from build123d import *

# Parameters (mm, degrees)
BOSS_EXTRUDE1_DEPTH     = 3
CUT_EXTRUDE4_DEPTH      = 13.469963913
CUT_EXTRUDE4_DEPTH_BACK = 13.469963913
CUT_EXTRUDE5_DEPTH      = 12.324751653
CUT_EXTRUDE5_DEPTH_BACK = 12.324751653
SKETCH6_R               = 18.5
FILLET1_R               = 0.5


with BuildPart() as part:
    # Sketch1 → Boss-Extrude1 (new, symmetric)
    with BuildSketch(Plane.XY):
        Polygon((-6, -1), (6, -1), (6, 1), (3.5, 1), (3.5, 7.5), (1.5, 7.5), (1.5, 1), (-1.5, 1), (-1.5, 7.5), (-3.5, 7.5), (-3.5, 1), (-6, 1), align=None)
    extrude(amount=BOSS_EXTRUDE1_DEPTH, both=True)

    # Sketch5 → Cut-Extrude4 (cut, two sides: drawn at the far end of the back side and taken through both)
    with BuildSketch(Plane.ZY.offset(3.5).offset(-CUT_EXTRUDE4_DEPTH_BACK)):
        with BuildLine():
            Line((1.25, 4.5), (-1.25, 4.5))
            ThreePointArc((-1.25, 4.5), (-2.25, 5.5), (-1.25, 6.5))
            Line((-1.25, 6.5), (1.25, 6.5))
            ThreePointArc((1.25, 6.5), (2.25, 5.5), (1.25, 4.5))
        make_face()
    extrude(amount=CUT_EXTRUDE4_DEPTH + CUT_EXTRUDE4_DEPTH_BACK, mode=Mode.SUBTRACT)

    # Sketch6 → Cut-Extrude5 (cut, two sides: drawn at the far end of the back side and taken through both)
    with BuildSketch(Plane.XY.offset(3).offset(-CUT_EXTRUDE5_DEPTH_BACK)):
        with Locations((0, -18.5)):
            Circle(SKETCH6_R)
        with BuildLine():
            Line((-6, 1), (-3.5, 1))
            ThreePointArc((-3.5, 1), (-4.760065757, 0.731270733), (-6, 0.381207588))
            Line((-6, 0.381207588), (-6, 1))
        make_face()
        with BuildLine():
            Line((3.5, 1), (6, 1))
            Line((6, 1), (6, 0.381207588))
            ThreePointArc((6, 0.381207588), (4.760065757, 0.731270733), (3.5, 1))
        make_face()
    extrude(amount=CUT_EXTRUDE5_DEPTH + CUT_EXTRUDE5_DEPTH_BACK, mode=Mode.SUBTRACT)

    # Fillet1
    fillet1_edges = [part.edges().sort_by_distance(p)[0] for p in [
        (6, -1, 0),
        (-6, -1, 0),
    ]]
    fillet(fillet1_edges, radius=FILLET1_R)


solid = part.part
Design review of the part built by this model. Coordinates are the model's own, in mm. A direction names the side the tool comes from. Coordinates: 2 decimals unless noted, no trailing zeros. Loops run counter-clockwise (first coordinate to the right, second up) from the corner with the lowest first, then second, coordinate; pieces in that order, holes last.
Item 1: Add section A-A (z = 0.15). Write out the cut boundary in (x, y), and give its area (3 significant figures).
Completed:
outline: (-6, -0.31) arc R0.5 ccw to (-5.36, -0.79) arc R18.5 cw to (5.36, -0.79) arc R0.5 ccw to (6, -0.31) - (6, 0.38) arc R19.81 ccw to (3.5, 1) - (3.5, 4.5) - (1.5, 4.5) - (1.5, 1) - (-1.5, 1) - (-1.5, 4.5) - (-3.5, 4.5) - (-3.5, 1) arc R19.81 ccw to (-6, 0.38) - close; (-3.5, 6.5) - (-1.5, 6.5) - (-1.5, 7.5) - (-3.5, 7.5) - close; (1.5, 6.5) - (3.5, 6.5) - (3.5, 7.5) - (1.5, 7.5) - close
area: 32.3 mm2
Item 2: Wall thickness on L1, parallel to X at y = 1.5, z = 2.1; L2, parallel to Y at x = -3.25, z = 1.95; L3, parallel to Y at x = -0.25, z = 2.65: over which ranges is each line inside the solid? List them lowest first.
Completed:
L1: x = -3.5 to -1.5, 1.5 to 3.5
L2: y = -0.29 to 4.79, 6.21 to 7.5
L3: y = 0 to 1
Item 3: Add section D-D (x = -2.5). Write out the cut boundary in (y, z).
Completed:
outline: (-0.17, -3) - (7.5, -3) - (7.5, 3) - (-0.17, 3) - close; hole (4.5, -1.25) arc R1 ccw to (6.5, -1.25) - (6.5, 1.25) arc R1 ccw to (4.5, 1.25) - close
Item 4: Clearance check with flat-ended pins moving along their axes: pin 1 (1.6 mm diameter, centred on x = 3, z = 0, fed in from -Y); pin 2 (1 mm diameter, centred on x = -2.5, z = 0.5, fed in from -Y); pin 3 (0.9 mm diameter, centred on x = 0.5, z = 1, fed in from +Y). State where each tip first meets the part, or that it passes through.
Completed:
pin 1: stops at y = -0.39
pin 2: stops at y = -0.24
pin 3: stops at y = 1
Item 5: Draft analysis for pull direction Z (two halves, no side actions). For faces 4 (the cylindrical face through (-2.49, 5.52, 2.25)), 5 (the flat face through (2, 2, 3)), 6 (the flat face through (-3.5, 4, 0)), state which applies: pulls with the +Z half, pulls with the -Z half, needs draft (parallel to the pull), parting line crosses it, or undercut.
Completed:
face 4: undercut
face 5: pulls with the +Z half
face 6: needs draft
Item 6: For faces 1 (the flat face through (0, 1, 0)), 2 (the flat face through (3.5, 3, 0)), 3 (the flat face through (3, 6.5, 0)), list the 3-axis set-ups (+Z, -Z, +X, -X, +Y, -Y) from which the entire face can be reached by the end or side of a thin tool; tool diameter is ignored.
Completed:
face 1: +Z, -Z, +Y
face 2: +Z, -Z, +X, +Y
face 3: +X, -X
Item 7: Add section B-B (y = 3). Write out the cut boundary in (x, z).
Completed:
outline: (-3.5, -3) - (-1.5, -3) - (-1.5, 3) - (-3.5, 3) - close; (1.5, -3) - (3.5, -3) - (3.5, 3) - (1.5, 3) - close
Item 8: Add section C-C (y = 5.5). Write out the cut boundary in (x, z), and give its area (3 significant figures).
Completed:
outline: (-3.5, -3) - (-1.5, -3) - (-1.5, -2.25) - (-3.5, -2.25) - close; (-3.5, 2.25) - (-1.5, 2.25) - (-1.5, 3) - (-3.5, 3) - close; (1.5, -3) - (3.5, -3) - (3.5, -2.25) - (1.5, -2.25) - close; (1.5, 2.25) - (3.5, 2.25) - (3.5, 3) - (1.5, 3) - close
area: 6.00 mm2
